Drawing for the job (mm, zero at the part's lowest x, y, z). A direction names the side the tool comes from. Coordinates: 2 decimals unless noted, no trailing zeros. Loops run counter-clockwise (first coordinate to the right, second up) from the corner with the lowest first, then second, coordinate; pieces in that order, holes last. Notation, with made-up numbers: (21.5, 7.25) -> (76.5, 7.25) arc R17 ccw to (76.5, 16.25) -> close; hole circle Ø8 at (84, 70.25). An arc over 180 degrees is marked (long way). Write item = value, one per line. Start each with the question number.
(1) Flat gauge pins, fed straight in: P1, Ø8, axis at y = 166.5, z = 297, coming from the +X side; P2, Ø10, axis at y = 291, z = 38, coming from the -X side; P3, Ø6, axis at y = 107, z = 145, coming from the +X side; P4, Ø5, axis at x = 60.5, z = 124, coming from the -Y side. Where does each tip first touch, or does it go through?
(2) Band-saw the part on B-B (y = 206). Write the cut outline in (x, z).
(3) Band-saw the part on A-A (z = 216). Write the cut outline in (x, y).
(4) Band-saw the part on D-D (y = 312). Write the cut outline in (x, z), and give its area (3 significant figures).
(5) Band-saw the part on C-C (x = 81). Write the cut outline in (y, z), and give its area (3 significant figures).
(6) Drill centre lines: line 1 (Y direction, x = 15.5, z = 171.5); line 2 (X direction, y = 307.5, z = 179); line 3 (X direction, y = 202, z = 124). Where is each one in solid material? Low to high. Write a range as from..to.
(7) Tool access for the marked faces 1 and 2: list every direction of +Z, -Z, +X, -X, +Y, -Y with a clear straight run to the whole face (end or side of a thin tool).
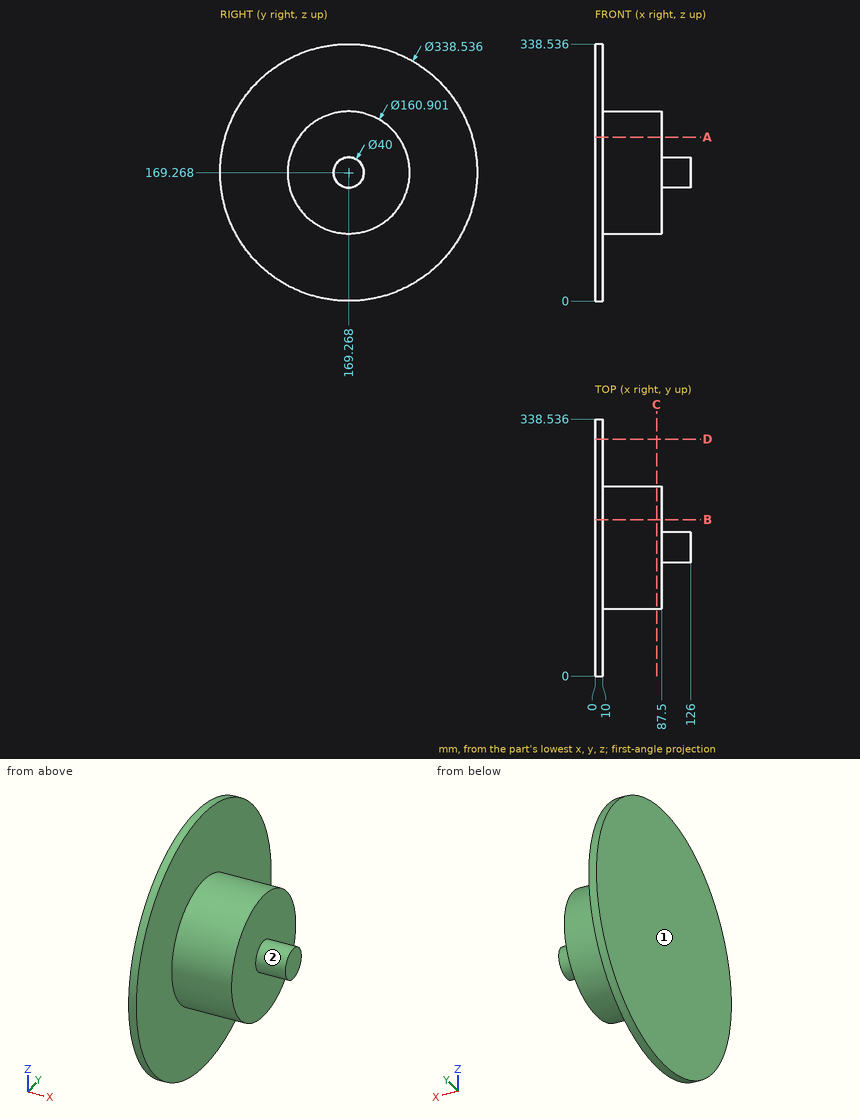
Findings below:
q1.P1 = 10
q1.P2 = through
q1.P3 = 87.5
q1.P4 = 101.13
q2.outline = (0, 4.03) -> (10, 4.03) -> (10, 97.69) -> (87.5, 97.69) -> (87.5, 240.84) -> (10, 240.84) -> (10, 334.5) -> (0, 334.5) -> close
q3.outline = (0, 6.58) -> (10, 6.58) -> (10, 103.78) -> (87.5, 103.78) -> (87.5, 234.75) -> (10, 234.75) -> (10, 331.96) -> (0, 331.96) -> close
q4.outline = (0, 78.28) -> (10, 78.28) -> (10, 260.26) -> (0, 260.26) -> close
q4.area = 1,820 mm²
q5.outline = circle Ø160.9 at (169.27, 169.27)
q5.area = 20,300 mm²
q6.line_1 = 88.85..249.69
q6.line_2 = 0..10
q6.line_3 = 0..87.5
q7.face_1 = +Z, -Z, -X, +Y, -Y
q7.face_2 = +X
